from build123d import *

# Parameters (mm, degrees)
SKETCH2_W          = 16
SKETCH2_H          = 10.5
BASE_DEPTH         = 2
ARM_DEPTH          = 2
LPATTERN1_COUNT    = 2
LPATTERN1_PITCH    = 14
SKETCH4_W          = 5
SKETCH4_H          = 5
CUT_EXTRUDE1_DEPTH = 34.4233972
FILLET1_R          = 2


with BuildPart() as part:
    # Sketch2 → base (new body)
    with BuildSketch(Plane(origin=(0, 0, 0), x_dir=(1, 0, 0), z_dir=(0, 1, 0))):
        Rectangle(SKETCH2_W, SKETCH2_H)
    extrude(amount=BASE_DEPTH)

    # Sketch3 → arm (add)
    with BuildSketch(Plane(origin=(8, 0, 0), x_dir=(0, 0, -1), z_dir=(1, 0, 0))):
        Polygon((5.25, 0), (5.25, 32), (-5.396617495, 32), (-5.396617495, 30), (1.201989129, 30), (-0.75, 0), align=None)
    arm = extrude(amount=-ARM_DEPTH)

    # LPattern1: arm ×2
    with Locations(*[(-i * LPATTERN1_PITCH, 0, 0) for i in range(1, LPATTERN1_COUNT)]):
        add(arm)

    # Sketch4 → Cut-Extrude1 (cut, through all)
    with BuildSketch(Plane.XZ):
        with Locations((0, -2.75)):
            Rectangle(SKETCH4_W, SKETCH4_H)
    extrude(amount=-CUT_EXTRUDE1_DEPTH, mode=Mode.SUBTRACT)

    # Fillet1
    fillet1_edges = [part.edges().sort_by_distance(p)[0] for p in [
        (2.5, 1, -0.25),
        (-2.5, 1, -0.25),
        (8, 1, 5.25),
        (-8, 1, 5.25),
    ]]
    fillet(fillet1_edges, radius=FILLET1_R)


solid = part.part
Design review of the part built by this model. Coordinates are the model's own, in mm. A direction names the side the tool comes from. Round coordinates to 2 decimals unless told otherwise and drop trailing zeros. Write each loop counter-clockwise with the first axis right and the second up, starting at its lowest first coordinate (ties: lowest second). Pieces come first, ordered by that corner, then holes. Notation, with made-up numbers: (58.25, 31) - (96.25, 31) arc R33 cw to (96.25, 60) - close; hole circle Ø2 at (77, 89.25). An arc over 180 degrees is marked (long way). Use a Markdown table: item, result. Add a question column.
1. We need section A-A (z = 1.5). State the section outline as (x, y) points, then the cut area to 3 significant figures.
2. We need section C-C (y = 23.5). State the section outline as (x, z) points.
3. Clearance check with flat-ended pins moving along their axes: pin 1 (6 mm diameter, centred on y = 26, z = 2.5, fed in from +X); pin 2 (2 mm diameter, centred on x = -2.5, y = 1, fed in from +Z); pin 3 (1 mm diameter, centred on x = 4.5, z = 1.5, fed in from +Y). State where each tip first meets the part, or that it passes through.
4. We need section D-D (z = -0.75). State the section outline as (x, y) points.
5. Wall thickness on probe 1 along X at (y, z) = (20, -3.75); probe 2 along Y at (x, z) = (1.25, 2); probe 3 along Z at (x, y) = (7.25, 27): over which ranges is each line inside the solid? List them lowest first.
6. Mouldability with a two-part tool opening along X and no side actions: class faces 1 (the face through (7.43, 1.01, 4.65)), 2 (the face through (2.5, 1, -4)), 3 (the face through (-6, 17, -2)), 4 (the face through (0, 1, 5.25)) as +X half, -X half, draft (parallel to the pull), parting line (faces both ways), or undercut.
7. We need section B-B (z = -3.5). State the section outline as (x, y) points.
8. For faces 5 (the face through (-7.43, 1.01, 4.65)), 6 (the face through (7, 30, 2)), 7 (the face through (6, 17, -2)), 8 (the face through (0, 2, 1)), list the 3-axis set-ups (+Z, -Z, +X, -X, +Y, -Y) from which the entire face can be reached by the end or side of a thin tool; tool diameter is ignored.
Output:
| question | item | result |
|---|---|---|
| 1 | outline | (-8, 0) - (8, 0) - (8, 2) - (-8, 2) - close; (-8, 30) - (-6, 30) - (-6, 32) - (-8, 32) - close; (6, 30) - (8, 30) - (8, 32) - (6, 32) - close |
| 1 | area | 40.0 mm2 |
| 2 | outline | (-8, -5.25) - (-6, -5.25) - (-6, -0.78) - (-8, -0.78) - close; (6, -5.25) - (8, -5.25) - (8, -0.78) - (6, -0.78) - close |
| 3 | pin 1 | passes through |
| 3 | pin 2 | stops at z = 5.25 |
| 3 | pin 3 | stops at y = 2 |
| 4 | outline | (-8, 0) - (-1.82, 0) - (-1.82, 2) - (-6, 2) - (-6, 23.05) - (-8, 23.05) - close; (-8, 30) - (-6, 30) - (-6, 32) - (-8, 32) - close; (1.82, 0) - (8, 0) - (8, 23.05) - (6, 23.05) - (6, 2) - (1.82, 2) - close; (6, 30) - (8, 30) - (8, 32) - (6, 32) - close |
| 5 | probe 1 | x = -8 to -6, 6 to 8 |
| 5 | probe 2 | y = 0 to 2 |
| 5 | probe 3 | z = -5.25 to -1.01 |
| 6 | face 1 | +X half |
| 6 | face 2 | undercut |
| 6 | face 3 | undercut |
| 6 | face 4 | draft |
| 7 | outline | (-8, 0) - (-2.5, 0) - (-2.5, 2) - (-6, 2) - (-6, 32) - (-8, 32) - close; (2.5, 0) - (8, 0) - (8, 32) - (6, 32) - (6, 2) - (2.5, 2) - close |
| 8 | face 5 | +Z, -X, -Y |
| 8 | face 6 | +Z, +X, -X |
| 8 | face 7 | +Z, -Z, +Y |
| 8 | face 8 | +Z |
